Verification items for the finished model (mm, model axes). Coordinates: 2 decimals unless noted, no trailing zeros. Loops run counter-clockwise (first coordinate to the right, second up) from the corner with the lowest first, then second, coordinate; pieces in that order, holes last. Notation, with made-up numbers: (74, -15.5) -> (132, -15.5) arc R34 ccw to (132, 17.5) -> close; hole circle Ø4 at (-4.5, -34). An arc over 180 degrees is marked (long way). Answer as a JSON object with one key per item and string values. Group by question number.
Q1. Gauge pin test, flat ends, axial feed: pin 1 Ø3 at (x, z) = (1.5, 2.5) entering from -Y; pin 2 Ø2 at (y, z) = (-2.5, -1.5) entering from +X; pin 3 Ø2 at (y, z) = (-2, -2) entering from -X. Record the tip position at first contact, or that the pin passes through.
Q2. Cross-section at A-A on y = -2.15. Record the boundary of the cut face in (x, z).
Q3. Scan lines: L1, parallel to Z at x = -1.1, y = -2.35; L2, parallel to Z at x = -0.9, y = -3.5; L3, parallel to X at y = -3.35, z = -2.5. Record each from-to range of solid material in increasing order.
Autodesk Inventor part; units mm, degrees
ref_plane "right_vertical_trmnls_XY" through (0, 0, 0) normal (0, 0, -1) x (1, 0, 0)
ref_plane "right_vertical_trmnls_YZ" through (0, 0, 0) normal (1, 0, 0) x (0, -1, 0)
ref_plane "right_vertical_trmnls_ZX" through (0, 0, 0) normal (0, -1, 0) x (0, 0, -1)
sketch "Sketch_1" plane through (0, 0, 0) normal (0, 1, 0) x (-1, 0, 0)
  line L0 (2.5146, 3.5052) -> (-2.5146, 3.5052)
  line L1 (-2.5146, 3.5052) -> (-2.5146, -3.5052)
  line L2 (-2.5146, -3.5052) -> (2.5146, -3.5052)
  line L3 (2.5146, -3.5052) -> (2.5146, 3.5052)
extrude "Extrusion1" add sketch "Sketch_1" along normal blind 0.0254
sketch "Sketch_2" plane through (0, 0, 0) normal (0, 1, 0) x (-1, 0, 0)
  circle A0 centre (0.9906, 0) radius 0.3048
extrude "Extrusion2" add sketch "Sketch_2" against normal blind 3.9624
sketch "Sketch_3" plane through (0, 0, 0) normal (0, 1, 0) x (-1, 0, 0)
  circle A0 centre (0.9906, -2.54) radius 0.3048
extrude "Extrusion3" add sketch "Sketch_3" against normal blind 3.9624
sketch "Sketch_4" plane through (0, 0, 0) normal (0, 1, 0) x (-1, 0, 0)
  circle A0 centre (0.9906, 2.54) radius 0.3048
extrude "Extrusion4" add sketch "Sketch_4" against normal blind 3.9624
ref_plane "right_vertical_trmnls_XY" through (0, 0, 0) normal (0, 0, -1) x (1, 0, 0)
ref_plane "right_vertical_trmnls_YZ" through (0, 0, 0) normal (1, 0, 0) x (0, -1, 0)
ref_plane "right_vertical_trmnls_ZX" through (0, 0, 0) normal (0, -1, 0) x (0, 0, -1)
ref_plane "stright_trmnls_XY" through (0, 0, 0) normal (0, -1, 0) x (1, 0, 0)
ref_plane "stright_trmnls_YZ" through (0, 0, 0) normal (1, 0, 0) x (0, 0, 1)
ref_plane "stright_trmnls_ZX" through (0, 0, 0) normal (0, 0, 1) x (0, -1, 0)
properties part number "B12APtrmnls"
Computed values:
{
 "1": {"pin 1": "stops at y = 0", "pin 2": "stops at x = -0.69", "pin 3": "stops at x = -1.3"},
 "2": {"outline": "circle Ø0.61 at (-0.99, -2.54); circle Ø0.61 at (-0.99, 0); circle Ø0.61 at (-0.99, 2.54)"},
 "3": {"L1": "z = -2.82 to -2.26, -0.28 to 0.28, 2.26 to 2.82", "L2": "z = -2.83 to -2.25, -0.29 to 0.29, 2.25 to 2.83", "L3": "x = -1.29 to -0.69"}
}
